Input: part model. Units: mm. Frame: model coordinates. A direction names the side the tool comes from. Give positions to 0.01 mm unless a question says otherwise; leave off trailing zeros. Use a Markdown table: item, result.
from build123d import *

# Parameters (mm, degrees)
F1_DEPTH = 30
F3_DEPTH = 150.001


with BuildPart() as f1:
    # F0 (on Top) → F1 (new body)
    with BuildSketch(Plane.XY):
        Polygon((-5, 23), (-7.5, 23), (-7.5, 0), (142.5, 0), (142.5, 23), (140, 23), (136.5, 3), (135, 3), (133.5, 3), (130, 23), (127.5, 23), (125, 23), (121.5, 3), (120, 3), (118.5, 3), (115, 23), (112.5, 23), (110, 23), (106.5, 3), (105, 3), (103.5, 3), (100, 23), (97.5, 23), (95, 23), (91.5, 3), (90, 3), (88.5, 3), (85, 23), (82.5, 23), (80, 23), (76.5, 3), (75, 3), (73.5, 3), (70, 23), (67.5, 23), (65, 23), (61.5, 3), (60, 3), (58.5, 3), (55, 23), (52.5, 23), (50, 23), (46.5, 3), (45, 3), (43.5, 3), (40, 23), (37.5, 23), (35, 23), (31.5, 3), (30, 3), (28.5, 3), (25, 23), (22.5, 23), (20, 23), (16.5, 3), (15, 3), (13.5, 3), (10, 23), (7.5, 23), (5, 23), (1.5, 3), (0, 3), (-1.5, 3), align=None)
    extrude(amount=F1_DEPTH)

    # F2 (on face) → F3 (cut, through all)
    with BuildSketch(Plane.YZ.offset(142.5)):
        Polygon((20, 28.908089), (23, 30), (0, 30), (0, 19.628685), (20, 26.908089), align=None)
        Polygon((23, 24.258563), (0, 0), (23, 0), align=None)
    extrude(amount=-F3_DEPTH, mode=Mode.SUBTRACT)


solid = f1.part
1. Material intervals for line 1 along Y through (x, z) = (104.5, 17); line 2 along Y through (x, z) = (112, 27.5); line 3 along Z through (x, y) = (23, 3), sorted ascending.
Response:
| item | result |
|---|---|
| line 1 | y = 0 to 3 |
| line 2 | y = 20 to 23 |
| line 3 | z = 3.16 to 20.72 |
2. Pin query (flat end, axial travel): pin 1 (1.6 mm diameter, centred on x = -5.5, z = 28, fed in from -Y); pin 2 (0.9 mm diameter, centred on x = 134.5, z = 11, fed in from +Y); pin 3 (12 mm diameter, centred on x = 118, y = 9, fed in from -Z). Return the tip coordinate at first contact, or that it passes through.
Response:
| item | result |
|---|---|
| pin 1 | stops at y = 20 |
| pin 2 | stops at y = 3 |
| pin 3 | stops at z = 3.16 |
3. Set-up query: faces 4 (the face through (135, 3, 12)), 5 (the face through (51.88, 7.64, 22.41)). Return all of +Z, -Z, +X, -X, +Y, -Y with unobstructed straight access to the full face (end or side cutting, diameter ignored); none if empty.
Response:
| item | result |
|---|---|
| face 4 | +Z, -Z, +Y |
| face 5 | +Z, +X, -X, -Y |
4. Mould query, pull axis X, two halves, no side actions, for faces 1 (the face through (141, 23, 27)), 2 (the face through (17.886, 10.918, 16.394)), 3 (the face through (-7.5, 9, 18)). Classes: pulls with the +X half, pulls with the -X half, needs draft (parallel to the pull), parting line crosses it, or undercut.
Response:
| item | result |
|---|---|
| face 1 | needs draft |
| face 2 | undercut |
| face 3 | pulls with the -X half |
5. Section query A-A (y = 4.75). State how many separate pieces and enclosed holes the cut face has, then the cut area to 3 significant figures.
Response:
| item | result |
|---|---|
| separate pieces | 11 |
| enclosed holes | 0 |
| area | 1,860 mm^2 |
